Could you check a few things on this model? Use its own coordinates, in mm. Face numbers are marked on the shaded views. Give positions to 0.01 mm unless a question says otherwise; leave off trailing zeros. Loops run counter-clockwise (first coordinate to the right, second up) from the corner with the lowest first, then second, coordinate; pieces in that order, holes last.
1. For P1, Ø2, axis at x = -15.72, z = 15.72, coming from the -Y side; P2, Ø23, axis at x = 0, z = 0, coming from the -Y side; P3, Ø1.4, axis at x = -15.72, z = 15.72, coming from the +Y side; P4, Ø12, axis at y = 85.5, z = 8, coming from the +X side, each with a flat end and sliding along its axis, tell me the tip position at first contact or that it passes through.
2. Imagine slicing it at B-B (z = 0). List the corners of the cut face in (x, y) for me.
3. Imagine slicing it at A-A (x = 0). List the corners of the cut face in (y, z) for me.
4. I need wall thicknesses on line 1 along Z through (x, y) = (0.5, 84.5); line 2 along X through (y, z) = (20, 0); line 3 along Z through (x, y) = (15, 10.5). Which ranges of each line are inside material? Lowest first, please.
5. Imagine slicing it at C-C (z = -8). List the corners of the cut face in (x, y) for me.
6. Imagine slicing it at D-D (y = 10). List the corners of the cut face in (x, z) for me.
7. Thinking about a two-plate mould opening in Z: for the marked faces 1, 2 and 3, which applies, +Z half, -Z half, draft (parallel to the pull), parting line (faces both ways), or undercut?
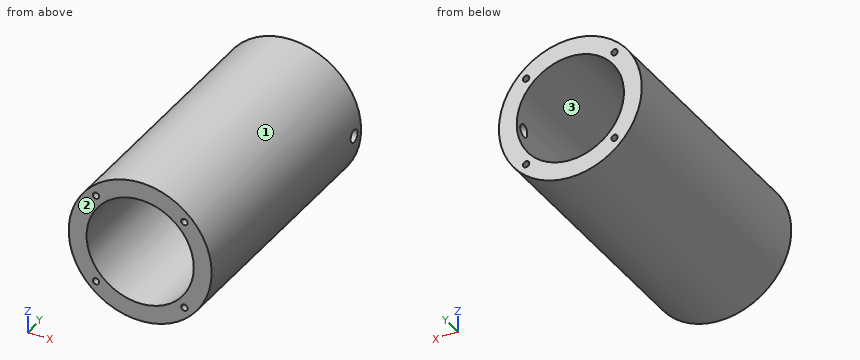
```python
from build123d import *

# Parameters (mm, degrees)
SKETCH1_R                      = 25.4
SKETCH1_R_2                    = 19.05
BOSS_EXTRUDE1_DEPTH            = 95.25
F_4_40_TAPPED_HOLE1_AT_2_COUNT = 2
F_4_40_TAPPED_HOLE1_AT_2_PITCH = 31.430896424
F_4_40_TAPPED_HOLE1_AT_3_COUNT = 2
F_4_40_TAPPED_HOLE1_AT_3_PITCH = 44.45
F_4_40_TAPPED_HOLE1_AT_4_COUNT = 2
F_4_40_TAPPED_HOLE1_AT_4_PITCH = 31.430896424
F_4_40_TAPPED_HOLE1_AT_5_COUNT = 2
F_4_40_TAPPED_HOLE1_AT_5_PITCH = 22.225
SKETCH7_W                      = 2.2479
SKETCH7_H                      = 25.4


with BuildPart() as part:
    # Sketch1 → Boss-Extrude1 (new body)
    with BuildSketch(Plane(origin=(0, 0, 0), x_dir=(1, 0, 0), z_dir=(0, 1, 0))):
        Circle(SKETCH1_R)
        Circle(SKETCH1_R_2, mode=Mode.SUBTRACT)
    extrude(amount=BOSS_EXTRUDE1_DEPTH)

    # Sketch2 → #4-40 Tapped Hole1 (revolve, cut)
    with BuildSketch(Plane(origin=(-15.715448212, 0, -15.715448212), x_dir=(0, 0, -1), z_dir=(1, 0, 0))):
        Polygon((0, 0), (0, 8.934152758), (1.1303, 8.255), (1.1303, 0), align=None)
    f_4_40_tapped_hole1 = revolve(axis=Axis((-15.715448212, -6.35, -15.715448212), (0, 1, 0)), mode=Mode.SUBTRACT)

    # #4-40 Tapped Hole1 at 2: #4-40 Tapped Hole1 ×2
    with Locations(*[(0, 0, i * F_4_40_TAPPED_HOLE1_AT_2_PITCH) for i in range(1, F_4_40_TAPPED_HOLE1_AT_2_COUNT)]):
        add(f_4_40_tapped_hole1, mode=Mode.SUBTRACT)

    # #4-40 Tapped Hole1 at 3: #4-40 Tapped Hole1 ×2
    with Locations(*[Vector(0.707106781, 0, 0.707106781) * (i * F_4_40_TAPPED_HOLE1_AT_3_PITCH) for i in range(1, F_4_40_TAPPED_HOLE1_AT_3_COUNT)]):
        add(f_4_40_tapped_hole1, mode=Mode.SUBTRACT)

    # #4-40 Tapped Hole1 at 4: #4-40 Tapped Hole1 ×2
    with Locations(*[(i * F_4_40_TAPPED_HOLE1_AT_4_PITCH, 0, 0) for i in range(1, F_4_40_TAPPED_HOLE1_AT_4_COUNT)]):
        add(f_4_40_tapped_hole1, mode=Mode.SUBTRACT)

    # #4-40 Tapped Hole1 at 5: #4-40 Tapped Hole1 ×2
    with Locations(*[Vector(0.707106781, 0, 0.707106781) * (i * F_4_40_TAPPED_HOLE1_AT_5_PITCH) for i in range(1, F_4_40_TAPPED_HOLE1_AT_5_COUNT)]):
        add(f_4_40_tapped_hole1, mode=Mode.SUBTRACT)

    # Mirror1: #4-40 Tapped Hole1 across plane
    add(f_4_40_tapped_hole1.mirror(Plane(origin=(0, 47.625, 0), x_dir=(0, 0, 1), z_dir=(0, -1, 0))), mode=Mode.SUBTRACT)

    # Mirror1 copy 1 sketch → Mirror1 copy 1 (revolve, cut)
    with BuildSketch(Plane(origin=(-15.715448212, 95.25, 15.715448212), x_dir=(0, 0, -1), z_dir=(1, 0, 0))):
        Polygon((0, 0), (0, -8.934152758), (1.1303, -8.255), (1.1303, 0), align=None)
    revolve(axis=Axis((-15.715448212, 101.6, 15.715448212), (0, 1, 0)), mode=Mode.SUBTRACT)

    # Mirror1 copy 2 sketch → Mirror1 copy 2 (revolve, cut)
    with BuildSketch(Plane(origin=(15.715448212, 95.25, 15.715448212), x_dir=(0, 0, -1), z_dir=(1, 0, 0))):
        Polygon((0, 0), (0, -8.934152758), (1.1303, -8.255), (1.1303, 0), align=None)
    revolve(axis=Axis((15.715448212, 101.6, 15.715448212), (0, 1, 0)), mode=Mode.SUBTRACT)

    # Mirror1 copy 3 sketch → Mirror1 copy 3 (revolve, cut)
    with BuildSketch(Plane(origin=(15.715448212, 95.25, -15.715448212), x_dir=(0, 0, -1), z_dir=(1, 0, 0))):
        Polygon((0, 0), (0, -8.934152758), (1.1303, -8.255), (1.1303, 0), align=None)
    revolve(axis=Axis((15.715448212, 101.6, -15.715448212), (0, 1, 0)), mode=Mode.SUBTRACT)

    # Mirror1 copy 4 sketch → Mirror1 copy 4 (revolve, cut)
    with BuildSketch(Plane(origin=(0, 95.25, 0), x_dir=(0, 0, -1), z_dir=(1, 0, 0))):
        Polygon((0, 0), (0, -8.934152758), (1.1303, -8.255), (1.1303, 0), align=None)
    revolve(axis=Axis((0, 101.6, 0), (0, 1, 0)), mode=Mode.SUBTRACT)

    # Sketch7 → #8 Clearance Hole1 (revolve, cut)
    with BuildSketch(Plane.ZX.offset(90.805)):
        with Locations((1.12395, 12.7)):
            Rectangle(SKETCH7_W, SKETCH7_H)
    revolve(axis=Axis((-6.35, 90.805, 0), (1, 0, 0)), mode=Mode.SUBTRACT)


solid = part.part
```
Derived:
1. P1: stops at y = 8.33
1. P2: passes through
1. P3: stops at y = 86.74
1. P4: stops at x = 25.32
2. outline: (-25.4, 0) - (-19.05, 0) - (-19.05, 95.25) - (-25.4, 95.25) - close; (19.05, 0) - (25.4, 0) - (25.4, 88.56) - (19.05, 88.56) - close; (19.05, 93.05) - (25.4, 93.05) - (25.4, 95.25) - (19.05, 95.25) - close
3. outline: (0, -25.4) - (95.25, -25.4) - (95.25, -19.05) - (0, -19.05) - close; (0, 19.05) - (95.25, 19.05) - (95.25, 25.4) - (0, 25.4) - close
4. line 1: z = -25.4 to -19.04, 19.04 to 25.4
4. line 2: x = -25.4 to -19.05, 19.05 to 25.4
4. line 3: z = -20.5 to -11.74, 11.74 to 20.5
5. outline: (-24.11, 0) - (-17.29, 0) - (-17.29, 95.25) - (-24.11, 95.25) - close; (17.29, 0) - (24.11, 0) - (24.11, 95.25) - (17.29, 95.25) - close
6. outline: circle Ø50.8 at (0, 0); hole circle Ø38.1 at (0, 0)
7. face 1: parting line
7. face 2: draft
7. face 3: undercut
